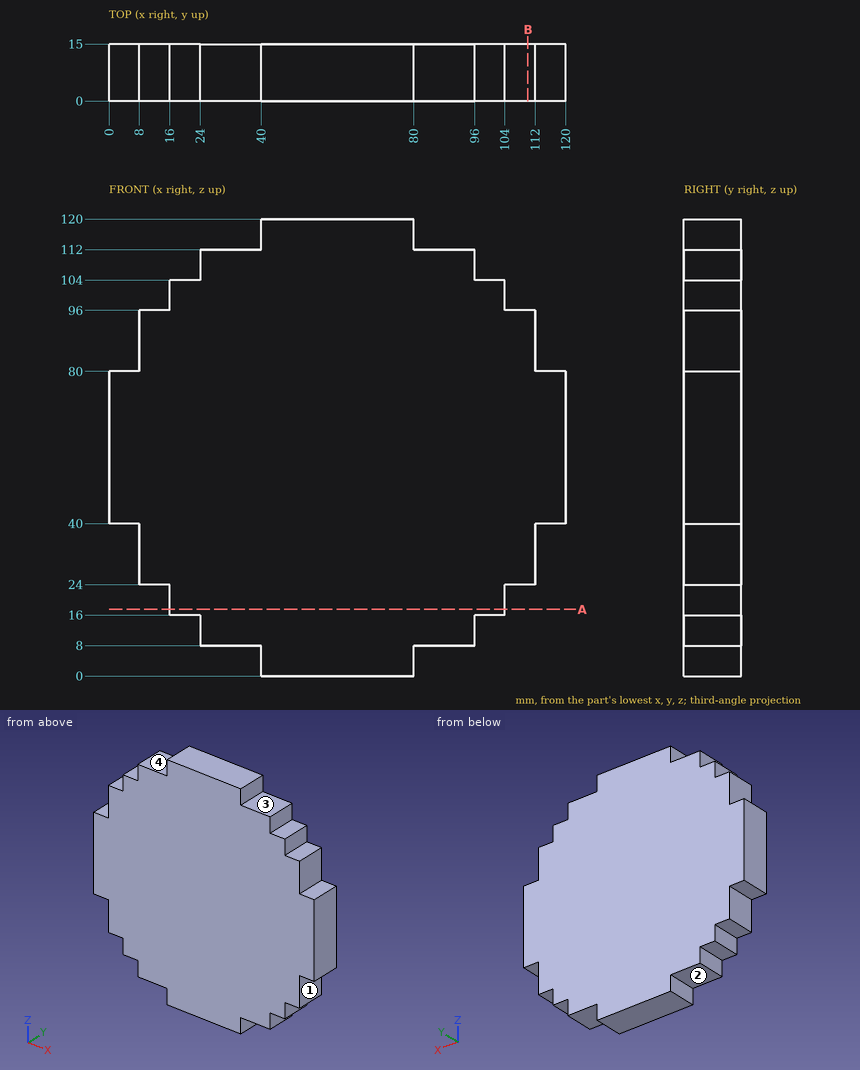
Geometry: see drawing. Coordinates: mm, zero at the bounding-box minimum. A direction names the side the tool comes from. Round coordinates to 2 decimals unless told otherwise and drop trailing zeros. Loops run counter-clockwise (first coordinate to the right, second up) from the corner with the lowest first, then second, coordinate; pieces in that order, holes last. Notation, with made-up numbers: (-28, 15) -> (8, 15) arc R19 cw to (8, 52) -> close; hole circle Ø8 at (49, 55). An arc over 180 degrees is marked (long way). Use one line per item in the form item = value. Start each with the question number.
Item 1: Section query A-A on z = 17.5. Return the cut outline in (x, y).
Item 2: Set-up query: the marked faces 1, 2, 3 and 4. Return all of +Z, -Z, +X, -X, +Y, -Y with unobstructed straight access to the full face (end or side cutting, diameter ignored); none if empty.
Item 3: Material intervals for L1, parallel to Z at x = 104.5, y = 1.25; L2, parallel to X at y = 1, z = 95.5, sorted ascending. Write a range as from..to.
Item 4: Contact query for flat-ended pins moving along their axis: pin 1 Ø4 at (y, z) = (11, 3.5) entering from +X; pin 2 Ø2.5 at (y, z) = (9, 3.5) entering from -X; pin 3 Ø4.5 at (x, y) = (86.5, 11) entering from +Z. Output: stop coordinate, or through.
Item 5: Section query B-B on x = 110. Return the cut outline in (y, z).
Ans:
q1.outline = (16, 0) -> (104, 0) -> (104, 15) -> (16, 15) -> close
q2.face_1 = -Z, +X, +Y, -Y
q2.face_2 = -Z, -X, +Y, -Y
q2.face_3 = +Z, +X, +Y, -Y
q2.face_4 = +Z, -X, +Y, -Y
q3.L1 = 24..96
q3.L2 = 8..112
q4.pin_1 = 80
q4.pin_2 = 40
q4.pin_3 = 112
q5.outline = (0, 24) -> (15, 24) -> (15, 96) -> (0, 96) -> close
